Geometry check sheet. Reference: the model listing, model coordinates, mm. Coordinates: 2 decimals unless noted, no trailing zeros. Loops run counter-clockwise (first coordinate to the right, second up) from the corner with the lowest first, then second, coordinate; pieces in that order, holes last.
from build123d import *

# Parameters (mm, degrees)
SKETCH1_R           = 39.9034
SKETCH1_R_2         = 38.1
BOSS_EXTRUDE1_DEPTH = 19.05
SKETCH2_R           = 6.1849
CUT_EXTRUDE1_DEPTH  = 57.431929465
SKETCH3_R           = 6.1849
CUT_EXTRUDE2_DEPTH  = 57.431929606


with BuildPart() as part:
    # Sketch1 → Boss-Extrude1 (new body, symmetric)
    with BuildSketch(Plane.XY):
        Circle(SKETCH1_R)
        Circle(SKETCH1_R_2, mode=Mode.SUBTRACT)
    extrude(amount=BOSS_EXTRUDE1_DEPTH, both=True)

    # Sketch2 → Cut-Extrude1 (cut, through all)
    with BuildSketch(Plane(origin=(0, 0, 0), x_dir=(0, 0, 1), z_dir=(-0.707106781, 0.707106781, 0))):
        with Locations((5.08, 0)):
            Circle(SKETCH2_R)
    extrude(amount=-CUT_EXTRUDE1_DEPTH, mode=Mode.SUBTRACT)

    # Sketch3 → Cut-Extrude2 (cut, through all)
    with BuildSketch(Plane(origin=(0, 0, 0), x_dir=(0, 0, 1), z_dir=(-0.707106781, -0.707106781, 0))):
        with Locations((5.08, 0)):
            Circle(SKETCH3_R)
    extrude(amount=CUT_EXTRUDE2_DEPTH, mode=Mode.SUBTRACT)


solid = part.part
1) Mould release check, pull along Y, two halves, no side actions. Record for faces 1 (the flat face through (32, -21, 19.05)), 2 (the cylindrical face through (38.06, 11.99, 0.27)), 3 (the cylindrical face through (36.34, 11.44, -0.27)), 4 (the cylindrical face through (23.51, -31.27, 7.93)): +Y half, -Y half, draft (parallel to the pull), parting line (faces both ways), or undercut.
Data:
face 1: draft
face 2: parting line
face 3: undercut
face 4: undercut
2) Material ranges on probe 1 along Y at (x, z) = (0, 13.5); probe 2 along Y at (x, z) = (9.5, -6.5); probe 3 along X at (y, z) = (-23, 13), recorded low to high.
Data:
probe 1: y = -39.9 to -38.1, 38.1 to 39.9
probe 2: y = -38.76 to -36.9, 36.9 to 38.76
probe 3: x = -32.61 to -30.37, 30.37 to 32.61
3) Depth check by flat-ended pin: pin 1 (2 mm diameter, centred on x = 0, z = 4, fed in from -Y); pin 2 (2 mm diameter, centred on y = 3.5, z = 4.5, fed in from -X) (3 decimals); pin 3 (12 mm diameter, centred on x = -20, z = 3.5, fed in from -Y); pin 4 (12 mm diameter, centred on x = 26, y = -25.5, fed in from -Z). Enter the tip coordinate at first touch or a pass-through.
Data:
pin 1: stops at y = -39.9
pin 2: stops at x = -39.825
pin 3: stops at y = -37.37
pin 4: stops at z = -19.05
4) Section check A-A on y = 0. Record the cut outline in (x, z).
Data:
outline: (-39.9, -19.05) - (-38.1, -19.05) - (-38.1, 19.05) - (-39.9, 19.05) - close; (38.1, -19.05) - (39.9, -19.05) - (39.9, 19.05) - (38.1, 19.05) - close
5) Section check D-D on x = -30. Count the separate pieces of the cut face and the enclosed holes in it, and give its area (3 significant figures).
Data:
separate pieces: 3
enclosed holes: 0
area: 187 mm2
6) Section check C-C on z = -10.5. Record the cut outline in (x, y).
Data:
outline: circle Ø79.81 at (0, 0); hole circle Ø76.2 at (0, 0)
